Part print with two shaded views. Sizes in mm from the minimum x, y, z corner. Give positions to 0.01 mm unless a question says otherwise; leave off trailing zeros. Order: outer loops, then holes, each group sorted by start corner. A loop starts at its lowest first (then second) coordinate and runs counter-clockwise, first axis right, second up. Notation, with made-up numbers: (33.25, 2) -> (39.25, 2) arc R20 ccw to (39.25, 8) -> close; hole circle Ø5 at (10, 42.5). An arc over 180 degrees is marked (long way). Answer as CSV lines item,"result".
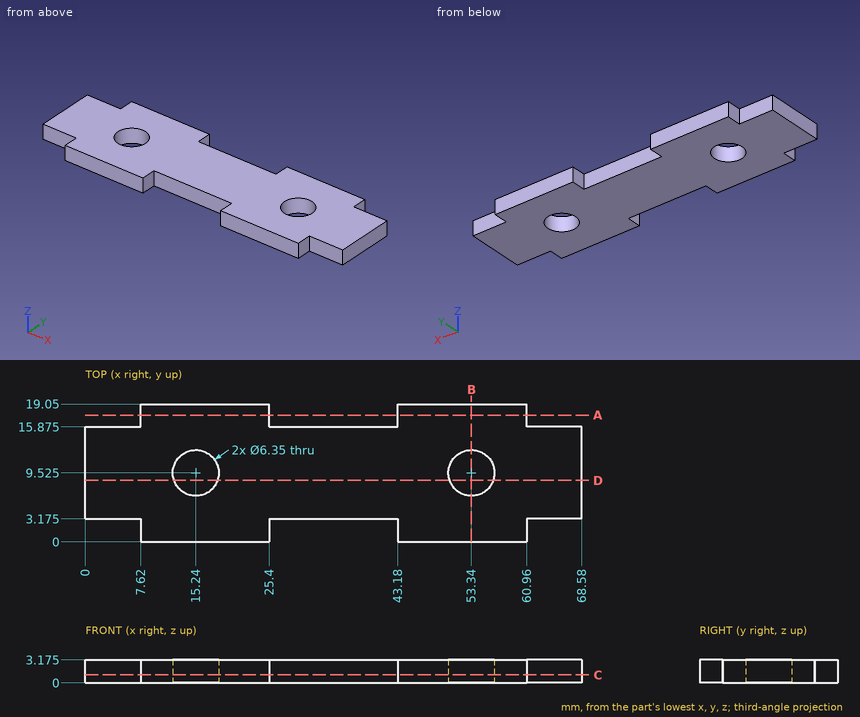
1) Band-saw the part on C-C, the plane z = 1.1. Write the cut outline in (x, y) (3 decimals).
Data:
outline,"(0, 3.175) -> (7.62, 3.175) -> (7.62, 0) -> (25.4, 0) -> (25.4, 3.175) -> (43.18, 3.175) -> (43.18, 0) -> (60.96, 0) -> (60.96, 3.175) -> (68.58, 3.175) -> (68.58, 15.875) -> (60.96, 15.875) -> (60.96, 19.05) -> (43.18, 19.05) -> (43.18, 15.875) -> (25.4, 15.875) -> (25.4, 19.05) -> (7.62, 19.05) -> (7.62, 15.875) -> (0, 15.875) -> close; hole circle Ø6.35 at (15.24, 9.525); hole circle Ø6.35 at (53.34, 9.525)"
2) Band-saw the part on B-B, the plane x = 53.34. Write the cut outline in (y, z) (3 decimals).
Data:
outline,"(0, 0) -> (6.35, 0) -> (6.35, 3.175) -> (0, 3.175) -> close; (12.7, 0) -> (19.05, 0) -> (19.05, 3.175) -> (12.7, 3.175) -> close"
3) Pin check, flat tips, straight feed: P1, Ø4, axis at x = 38.5, y = 2.5, coming from the -Z side; P2, Ø1.6, axis at y = 17, z = 1.5, coming from the +X side; P3, Ø1.6, axis at x = 33.5, z = 1, coming from the +Y side (3 decimals); P4, Ø1.6, axis at x = 63.5, z = 1.5, coming from the -Y side (3 decimals). Stop position of each tip, or through.
Data:
P1,"stops at z = 0"
P2,"stops at x = 60.96"
P3,"stops at y = 15.875"
P4,"stops at y = 3.175"
4) Wall check: line 1 along X through (y, z) = (2, 2.2); line 2 along X through (y, z) = (7.5, 0.75); line 3 along X through (y, z) = (7.25, 0.8). Give the ranges that are in metal, low to high. Write a range as [from, to].
Data:
line 1,"x = [7.62, 25.4], [43.18, 60.96]"
line 2,"x = [0, 12.79], [17.69, 50.89], [55.79, 68.58]"
line 3,"x = [0, 13.03], [17.45, 51.13], [55.55, 68.58]"
5) Band-saw the part on A-A, the plane y = 17.5. Write the cut outline in (x, z) (3 decimals), then the cut area to 3 significant figures.
Data:
outline,"(7.62, 0) -> (25.4, 0) -> (25.4, 3.175) -> (7.62, 3.175) -> close; (43.18, 0) -> (60.96, 0) -> (60.96, 3.175) -> (43.18, 3.175) -> close"
area,"113 mm2"
6) Band-saw the part on D-D, the plane y = 8.5. Write the cut outline in (x, z) (3 decimals).
Data:
outline,"(0, 0) -> (12.235, 0) -> (12.235, 3.175) -> (0, 3.175) -> close; (18.245, 0) -> (50.335, 0) -> (50.335, 3.175) -> (18.245, 3.175) -> close; (56.345, 0) -> (68.58, 0) -> (68.58, 3.175) -> (56.345, 3.175) -> close"
